```python
from build123d import *

# Parameters (mm, degrees)
BOSS_EXTRUDE1_DEPTH = 5
CUT_EXTRUDE1_DEPTH  = 50


with BuildPart() as part:
    # Sketch1 → Boss-Extrude1 (new, symmetric)
    with BuildSketch(Plane(origin=(0, 0, 0), x_dir=(1, 0, 0), z_dir=(0, 1, 0))):
        Polygon((0, 0), (-23, 0), (-23, -60), (-13, -60), (-13, -10), (0, -10), align=None)
    extrude(amount=BOSS_EXTRUDE1_DEPTH, both=True)

    # Sketch2 → Cut-Extrude1 (cut)
    with BuildSketch(Plane.XY.offset(60)):
        Polygon((-13, 5), (-23, 5), (-13, 0), align=None)
        Polygon((-13, -5), (-13, 0), (-23, -5), align=None)
    extrude(amount=-CUT_EXTRUDE1_DEPTH, mode=Mode.SUBTRACT)


solid = part.part
```
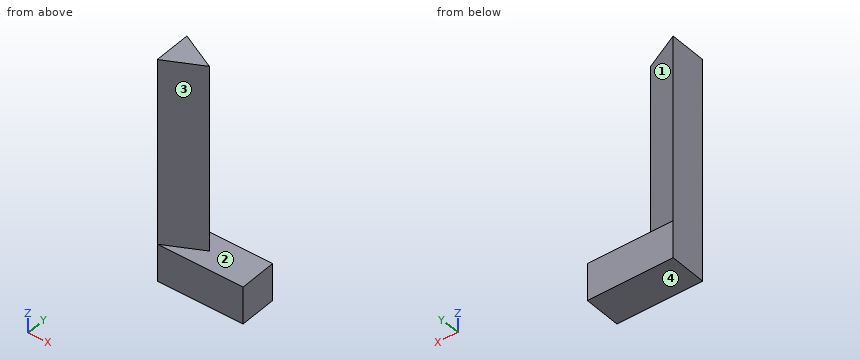
Geometry check sheet. Reference: the model listing, model coordinates, mm. Face numbers are marked on the shaded views. A direction names the side the tool comes from. Give positions to 0.01 mm unless a question says otherwise; leave off trailing zeros. Loops run counter-clockwise (first coordinate to the right, second up) from the corner with the lowest first, then second, coordinate; pieces in that order, holes last. Notation, with made-up numbers: M -16,-4.75 L -12,-4.75 A19 ccw -12,15.25 Z; hole C 47,71.5 d4. An arc over 180 degrees is marked long. Write item = value, one per line. Start each with the question number.
1. Section check A-A, the plane y = -2. Enter the section's corners in (x, z), plus the area to 3 significant figures.
2. Section check C-C, the plane y = 1. Enter the section's corners in (x, z), plus the area to 3 significant figures.
3. Section check B-B, the plane x = -17.25. Enter the section's corners in (y, z) (3 decimals).
4. Go/stop test with flat-tipped pins: P1, Ø3, axis at y = -2, z = 25.5, coming from the +X side; P2, Ø5, axis at x = -7.5, y = 0, coming from the +Z side. Record where each tip stops, or that it passes through.
5. Thickness scan on probe 1 along Z at (x, y) = (-9, 3); probe 2 along Y at (x, z) = (-13.75, 15) (3 decimals); probe 3 along X at (y, z) = (0.5, 28). Record the ranges inside material, lowest first.
6. Section check D-D, the plane z = 43.5. Enter the section's corners in (x, y), plus the area to 3 significant figures.
7. Tool access check on the marked faces 1, 2, 3 and 4. Record the directions out of +Z, -Z, +X, -X, +Y, -Y that give a thin tool (end or side, any length) a straight path to the whole face; none if there is none.
Values follow:
q1.outline = M -23,0 L 0,0 L 0,10 L -17,10 L -17,60 L -23,60 Z
q1.area = 530 mm^2
q2.outline = M -23,0 L 0,0 L 0,10 L -15,10 L -15,60 L -23,60 Z
q2.area = 630 mm^2
q3.outline = M -5,0 L 5,0 L 5,10 L 2.125,10 L 2.125,60 L -2.125,60 L -2.125,10 L -5,10 Z
q4.P1 = -14
q4.P2 = 10
q5.probe_1 = 0 to 10
q5.probe_2 = -0.375 to 0.375
q5.probe_3 = -23 to -14
q6.outline = M -23,-5 L -13,0 L -23,5 Z
q6.area = 50.0 mm^2
q7.face_1 = +Z, +X, +Y
q7.face_2 = +Z, +X
q7.face_3 = +Z, +X, -Y
q7.face_4 = -Z, +X, -X, +Y, -Y
